Model file for the job. Use its own axes, mm. Face numbers are marked on the shaded views. A direction names the side the tool comes from. Round coordinates to 2 decimals unless told otherwise and drop trailing zeros. Order: outer loops, then holes, each group sorted by start corner. A loop starts at its lowest first (then second) coordinate and runs counter-clockwise, first axis right, second up. Notation, with made-up numbers: (61.25, 30.5) -> (86.25, 30.5) arc R18 ccw to (86.25, 45.5) -> close; hole circle Ø6 at (-39, -16.5). An arc over 180 degrees is marked (long way). Put each result on its own line as item: value. Start each with the question number.
Q1. Flat gauge pins, fed straight in: P1, Ø10, axis at x = 31, z = -86.5, coming from the +Y side; P2, Ø16, axis at x = 110.5, y = 53, coming from the +Z side; P3, Ø3, axis at x = 67.5, y = 35, coming from the +Z side. Where does each tip first touch, or does it go through?
Q2. Cut at A-A, the plane z = -63.5. List the corners of the cut face in (x, y), and give its area (3 significant figures).
Q3. Cut at C-C, the plane y = 64.5. List the corners of the cut face in (x, z), and give its area (3 significant figures).
Q4. Probe L1, parallel to Z at x = 57.5, y = 10; L2, parallel to Z at x = 14.5, y = 66; L3, parallel to Y at x = 14, z = -29. List the from-to ranges inside material, lowest first.
Q5. 3-axis set-ups, long thin cutter, end or side, ignore diameter. For the marked faces 1, 2 and 3: which of +Z, -Z, +X, -X, +Y, -Y reach the whole face in a straight line?
Q6. Cut at D-D, the plane z = -44. List the corners of the cut face in (x, y).
Q7. Cut at B-B, the plane x = 7.5. List the corners of the cut face in (y, z), and give its area (3 significant figures).
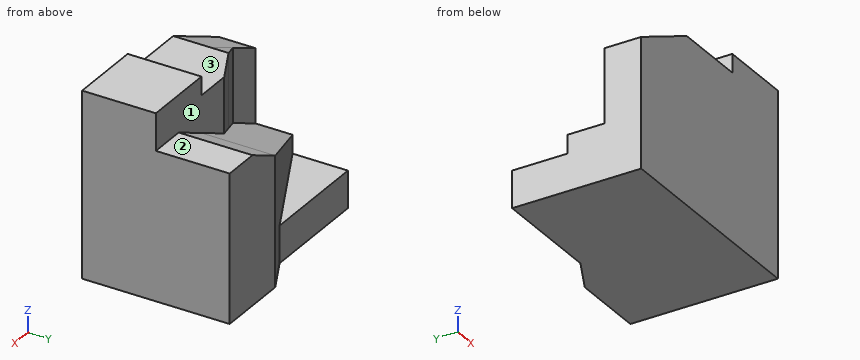
from build123d import *

# Parameters (mm, degrees)
SKETCH1_W            = 120
SKETCH1_H            = 100
BOSS_EXTRUDE1_DEPTH  = 20
CUT_EXTRUDE1_DEPTH   = 20
SKETCH3_W            = 40
SKETCH3_H            = 40
BOSS_EXTRUDE3_DEPTH  = 100
BOSS_EXTRUDE4_DEPTH  = 90
SKETCH5_W            = 20
SKETCH5_H            = 40
BOSS_EXTRUDE6_DEPTH  = 80
BOSS_EXTRUDE7_DEPTH  = 80
SKETCH7_W            = 60
SKETCH7_H            = 50
BOSS_EXTRUDE8_DEPTH  = 20
SKETCH8_W            = 10
SKETCH8_H            = 20
BOSS_EXTRUDE9_DEPTH  = 10
BOSS_EXTRUDE10_DEPTH = 42
BOSS_EXTRUDE18_DEPTH = 42
BOSS_EXTRUDE19_DEPTH = 30
BOSS_EXTRUDE21_DEPTH = 30
BOSS_EXTRUDE22_DEPTH = 30
BOSS_EXTRUDE23_DEPTH = 30
BOSS_EXTRUDE24_DEPTH = 30
SKETCH22_W           = 120
SKETCH22_H           = 100
CUT_EXTRUDE3_DEPTH   = 30


with BuildPart() as part:
    # Sketch1 → Boss-Extrude1 (new body)
    with BuildSketch(Plane(origin=(0, 0, 0), x_dir=(1, 0, 0), z_dir=(0, 1, 0))):
        with Locations((60, 50)):
            Rectangle(SKETCH1_W, SKETCH1_H)
    extrude(amount=BOSS_EXTRUDE1_DEPTH)

    # Sketch2 → Cut-Extrude1 (cut)
    with BuildSketch(Plane(origin=(0, 20, 0), x_dir=(1, 0, 0), z_dir=(0, 1, 0))):
        Polygon((0, 30), (40, 10), (80, 10), (80, 0), (0, 0), align=None)
    extrude(amount=-CUT_EXTRUDE1_DEPTH, mode=Mode.SUBTRACT)

    # Sketch3 → Boss-Extrude3 (add)
    with BuildSketch(Plane.XY):
        with Locations((100, 20)):
            Rectangle(SKETCH3_W, SKETCH3_H)
    extrude(amount=-BOSS_EXTRUDE3_DEPTH)

    # Sketch4 → Boss-Extrude4 (add)
    with BuildSketch(Plane.XY.offset(-10)):
        Polygon((80, 20), (80, 40), (60, 40), (40, 30), (40, 20), align=None)
    extrude(amount=-BOSS_EXTRUDE4_DEPTH)

    # Sketch5 → Boss-Extrude6 (add)
    with BuildSketch(Plane.XY.offset(-20)):
        with Locations((110, 60)):
            Rectangle(SKETCH5_W, SKETCH5_H)
    extrude(amount=-BOSS_EXTRUDE6_DEPTH)

    # Sketch6 → Boss-Extrude7 (add)
    with BuildSketch(Plane(origin=(0, 80, 0), x_dir=(1, 0, 0), z_dir=(0, 1, 0))):
        Polygon((100, 100), (80, 100), (80, 30), (100, 20), align=None)
    extrude(amount=-BOSS_EXTRUDE7_DEPTH)

    # Sketch7 → Boss-Extrude8 (add)
    with BuildSketch(Plane(origin=(0, 0, -100), x_dir=(-1, 0, 0), z_dir=(0, 0, -1))):
        with Locations((-30, 45)):
            Rectangle(SKETCH7_W, SKETCH7_H)
    extrude(amount=-BOSS_EXTRUDE8_DEPTH)

    # Sketch8 → Boss-Extrude9 (add)
    with BuildSketch(Plane.XY.offset(-80)):
        with Locations((5, 30)):
            Rectangle(SKETCH8_W, SKETCH8_H)
    extrude(amount=BOSS_EXTRUDE9_DEPTH)

    # Sketch9 → Boss-Extrude10 (add)
    with BuildSketch(Plane(origin=(-16, 32, 0), x_dir=(-0.894427191, -0.447213595, 0), z_dir=(0.447213595, -0.894427191, 0))):
        Polygon((-107.33126292, 100), (-107.33126292, 30), (-17.88854382, 70), (-17.88854382, 80), align=None)
    extrude(amount=BOSS_EXTRUDE10_DEPTH)

    # Sketch11 → Boss-Extrude18 (add)
    with BuildSketch(Plane(origin=(0, 0, -100), x_dir=(-1, 0, 0), z_dir=(0, 0, -1))):
        Polygon((-80, 40), (-60, 40), (-60, 70), (-80, 80), align=None)
    extrude(amount=-BOSS_EXTRUDE18_DEPTH)

    # Sketch12 → Boss-Extrude19 (add)
    with BuildSketch(Plane(origin=(28, 0, -56), x_dir=(0.894427191, 0, 0.447213595), z_dir=(-0.447213595, 0, 0.894427191))):
        Polygon((58.137767415, 80), (58.137767415, 40), (-31.304951685, 20), (-31.304951685, 40), align=None)
    extrude(amount=-BOSS_EXTRUDE19_DEPTH)

    # Sketch17 → Boss-Extrude21 (add)
    with BuildSketch(Plane(origin=(28, 0, -56), x_dir=(0.894427191, 0, 0.447213595), z_dir=(-0.447213595, 0, 0.894427191))):
        Polygon((13.416407865, 30), (-31.304951685, 20), (13.416407865, 20), align=None)
    extrude(amount=-BOSS_EXTRUDE21_DEPTH)

    # Sketch19 → Boss-Extrude22 (add)
    with BuildSketch(Plane(origin=(-4, 8, 0), x_dir=(0.894427191, 0.447213595, 0), z_dir=(-0.447213595, 0.894427191, 0))):
        Polygon((26.83281573, 20), (71.55417528, 10), (71.55417528, 40), (26.83281573, 60), align=None)
    extrude(amount=-BOSS_EXTRUDE22_DEPTH)

    # Sketch20 → Boss-Extrude23 (add)
    with BuildSketch(Plane(origin=(-4, 8, 0), x_dir=(0.894427191, 0.447213595, 0), z_dir=(-0.447213595, 0.894427191, 0))):
        Polygon((49.193495505, 10), (26.83281573, 20), (49.193495505, 15), align=None)
    extrude(amount=-BOSS_EXTRUDE23_DEPTH)

    # Sketch21 → Boss-Extrude24 (add)
    with BuildSketch(Plane(origin=(12, 0, -24), x_dir=(0.894427191, 0, 0.447213595), z_dir=(-0.447213595, 0, 0.894427191))):
        Polygon((8.94427191, 20), (31.304951685, 30), (31.304951685, 20), align=None)
    extrude(amount=-BOSS_EXTRUDE24_DEPTH)

    # Sketch22 → Cut-Extrude3 (cut)
    with BuildSketch(Plane.XZ):
        with Locations((60, -50)):
            Rectangle(SKETCH22_W, SKETCH22_H)
    extrude(amount=CUT_EXTRUDE3_DEPTH, mode=Mode.SUBTRACT)


solid = part.part
Ans:
1. P1: stops at y = 70
1. P2: stops at z = -20
1. P3: stops at z = -10
2. outline: (0, 0) -> (120, 0) -> (120, 80) -> (80, 80) -> (13, 46.5) -> (13, 20) -> (0, 20) -> close
2. area: 7,700 mm^2
3. outline: (0, -100) -> (120, -100) -> (120, -20) -> (100, -20) -> (49, -45.5) -> (49, -80) -> (0, -80) -> close
3. area: 6,010 mm^2
4. L1: z = -100 to -10
4. L2: z = -100 to -80
4. L3: y = 0 to 20
5. face 1: +Z, -X, +Y
5. face 2: +Z, +X, -X, +Y
5. face 3: +Z, -X, +Y, -Y
6. outline: (0, 0) -> (120, 0) -> (120, 80) -> (80, 80) -> (52, 66) -> (52, 36) -> (20, 20) -> (0, 20) -> close
7. outline: (0, -100) -> (70, -100) -> (70, -80) -> (43.75, -80) -> (43.75, -66.25) -> (20, -66.25) -> (20, -26.25) -> (0, -26.25) -> close
7. area: 2,800 mm^2
